Read the model definition and answer for the solid it produces. Units are mm, in the model's axes. Round coordinates to 2 decimals unless told otherwise and drop trailing zeros. Write each loop counter-clockwise with the first axis right and the second up, starting at its lowest first coordinate (ties: lowest second). Pieces come first, ordered by that corner, then holes. Notation, with made-up numbers: (-32, 45.5) -> (-19, 45.5) arc R27 ccw to (-19, 80.5) -> close; hole circle Ø11 at (47, 46). An arc over 180 degrees is marked (long way). Return JSON: item names as keys, results as strings. Group by question number.
(1) A cutting plane is placed at C-C on x = -20. Give the vertices of the cut face in (y, z), then the cut area to 3 significant figures.
(2) A cutting plane is placed at B-B on y = 0. Give the vertices of the cut face in (x, z), then the cut area to 3 significant figures.
(3) A cutting plane is placed at D-D on y = 3.5. Give the vertices of the cut face in (x, z).
(4) Given pin 1 (2.5 mm diameter, centred on x = -20, y = 0, fed in from -Z); pin 2 (5 mm diameter, centred on x = 20, y = 0, fed in from -Z), each flat-ended and moving along its own axis, determine where each tip first touches the part or whether it passes through.
(5) The mould has two halves that part along X. Classify faces 1 (the cylindrical face through (-21.5, 0.07, 1.48)), 2 (the flat face through (-19.947, -6.157, 1.479)), 3 (the flat face through (20.03, -6.1, 1.48)): released by +X, released by -X, zero draft, split by the parting line, or undercut.
(6) A cutting plane is placed at A-A on z = 0.8. Give the vertices of the cut face in (x, y).
(7) Straight lines are drawn through the part: line 1 (Y direction, x = -20, z = 1.95); line 2 (X direction, y = -0.5, z = 2.65); line 3 (X direction, y = -0.75, z = 0.4). For each, find the intervals that lie inside material, in ascending order.
```python
from build123d import *

# Parameters (mm, degrees)
ESBO_O1_R                = 1.5
ESBO_O1_W                = 29
ESBO_O1_H                = 20
RESSALTO_EXTRUS_O1_DEPTH = 3
FILETE1_R                = 10


with BuildPart() as part:
    # Esboço1 → Ressalto-extrusão1 (new body)
    with BuildSketch(Plane.XY):
        with BuildLine():
            Line((-22.882588201, 4.085423511), (-14.5, 10))
            Line((-14.5, 10), (-14.5, -10))
            Line((-14.5, -10), (-22.882588201, -4.085423511))
            ThreePointArc((-22.882588201, -4.085423511), (-25, 0), (-22.882588201, 4.085423511))
        make_face()
        with Locations((-20, 0)):
            Circle(ESBO_O1_R, mode=Mode.SUBTRACT)
        Rectangle(ESBO_O1_W, ESBO_O1_H)
        with BuildLine():
            ThreePointArc((22.882588201, 4.085423511), (25, 0), (22.882588201, -4.085423511))
            Line((22.882588201, -4.085423511), (14.5, -10))
            Line((14.5, -10), (14.5, 10))
            Line((14.5, 10), (22.882588201, 4.085423511))
        make_face()
        with Locations((20, 0)):
            Circle(ESBO_O1_R, mode=Mode.SUBTRACT)
    extrude(amount=RESSALTO_EXTRUS_O1_DEPTH)

    # Filete1
    filete1_edges = [part.edges().sort_by_distance(p)[0] for p in [
        (-14.5, 10, 1.5),
        (14.5, 10, 1.5),
        (14.5, -10, 1.5),
        (-14.5, -10, 1.5),
    ]]
    fillet(filete1_edges, radius=FILETE1_R)


solid = part.part
```
Checks:
{
 "1": {"outline": "(-6.12, 0) -> (-1.5, 0) -> (-1.5, 3) -> (-6.12, 3) -> close; (1.5, 0) -> (6.12, 0) -> (6.12, 3) -> (1.5, 3) -> close", "area": "27.7 mm^2"},
 "2": {"outline": "(-25, 0) -> (-21.5, 0) -> (-21.5, 3) -> (-25, 3) -> close; (-18.5, 0) -> (18.5, 0) -> (18.5, 3) -> (-18.5, 3) -> close; (21.5, 0) -> (25, 0) -> (25, 3) -> (21.5, 3) -> close", "area": "132 mm^2"},
 "3": {"outline": "(-23.57, 0) -> (23.57, 0) -> (23.57, 3) -> (-23.57, 3) -> close"},
 "4": {"pin 1": "passes through", "pin 2": "stops at z = 0"},
 "5": {"face 1": "undercut", "face 2": "released by -X", "face 3": "released by +X"},
 "6": {"outline": "(-22.88, -4.09) -> (-17.09, -8.17) arc R10 ccw to (-11.33, -10) -> (11.33, -10) arc R10 ccw to (17.09, -8.17) -> (22.88, -4.09) arc R5 ccw to (22.88, 4.09) -> (17.09, 8.17) arc R10 ccw to (11.33, 10) -> (-11.33, 10) arc R10 ccw to (-17.09, 8.17) -> (-22.88, 4.09) arc R5 ccw to start; hole circle Ø3 at (-20, 0); hole circle Ø3 at (20, 0)"},
 "7": {"line 1": "y = -6.12 to -1.5, 1.5 to 6.12", "line 2": "x = -24.97 to -21.41, -18.59 to 18.59, 21.41 to 24.97", "line 3": "x = -24.94 to -21.3, -18.7 to 18.7, 21.3 to 24.94"}
}
